The listing builds one solid part. Answer for the finished solid, in the listing's coordinates (mm). Face numbers are marked on the shaded views. A direction names the side the tool comes from. Give positions to 0.01 mm unless a question says otherwise; leave off trailing zeros. Write each loop counter-clockwise with the first axis right and the second up, starting at its lowest first coordinate (ties: lowest second). Pieces come first, ordered by that corner, then holes. Notation, with made-up numbers: (70.25, -32.5) - (113.25, -32.5) arc R21 cw to (113.25, -15.5) - close; hole circle Ø2 at (3.25, 56). An arc over 180 degrees is marked (long way). Answer as CSV lines item,"result". Start each with the question number.
(1) Find section B-B (x = -22). Write down the section's boundary in (y, z).
(2) Find section C-C (x = 102). Write down the section's boundary in (y, z).
(3) Find section A-A (y = -1079.5). Write down the section's boundary in (x, z).
(4) Straight lines are drawn through the part: probe 1 along Y at (x, z) = (-187.5, 29); probe 2 along Y at (x, z) = (-298, 49); probe 3 along Y at (x, z) = (-159, 67). For each, find the intervals that lie inside material, in ascending order.
(5) For a pull along X with two mould halves and no side action, classify the marked faces 3, 4 and 5 as pulls with the +X half, pulls with the -X half, needs draft (parallel to the pull), parting line crosses it, or undercut.
(6) Each of these flat-tipped pins is pushed along its axis until it touches: pin 1 Ø3 at (x, z) = (25, 78) entering from +Y; pin 2 Ø1.5 at (y, z) = (-348, 79) entering from -X; pin 3 Ø4 at (x, z) = (-44.5, 26) entering from +Y. Where does it stop, or does it pass through?
(7) For the marked faces 1 and 2, determine the directions among +Z, -Z, +X, -X, +Y, -Y from which every point of the face is accessible in a straight line to the end or side of a thin tool.
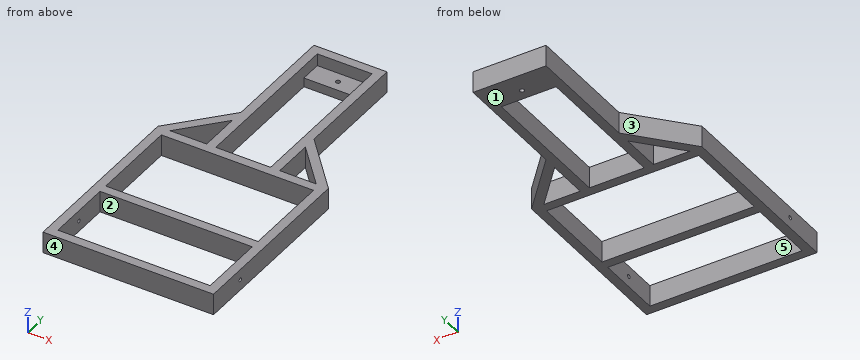
from build123d import *

# Parameters (mm, degrees)
F0_W          = 635
F0_H          = 38.1
F0_W_2        = 38.1
F1_DEPTH      = 88.9
F0_W_3        = 228.6
F0_H_2        = 88.9
F2_DEPTH      = 38.1
F3_R          = 9.525
F4_DEPTH      = 38.101
F5_R          = 7.9375
F6_DEPTH      = 673.101
F6_DEPTH_BACK = 38.101


with BuildPart() as f1:
    # F0 (on Top) → F1 (new body)
    with BuildSketch(Plane.XY):
        Polygon((0, -484.015493486), (0, 0), (-304.8, 0), (-304.8, -484.015493486), (-304.8, -541.165493486), (-304.8, -711.2), (-266.7, -711.2), (-266.7, -127), (-266.7, -38.1), (-38.1, -38.1), (-38.1, -127), (-38.1, -711.2), (0, -711.2), (0, -541.165493486), align=None)
        Polygon((-304.8, -541.165493486), (-304.8, -484.015493486), (-508, -711.2), (-456.8834860344, -711.2), align=None)
        Polygon((203.2, -711.2), (0, -484.015493486), (0, -541.165493486), (152.0834860344, -711.2), align=None)
        Polygon((203.2, -1117.6), (203.2, -711.2), (152.0834860344, -711.2), (0, -711.2), (-38.1, -711.2), (-152.4, -711.2), (-266.7, -711.2), (-304.8, -711.2), (-456.8834860344, -711.2), (-508, -711.2), (-508, -1117.6), (-469.9, -1117.6), (-469.9, -749.3), (165.1, -749.3), (165.1, -1117.6), align=None)
        with Locations((-152.4, -1136.65)):
            Rectangle(F0_W, F0_H)
        with Locations((184.15, -1136.65)):
            Rectangle(F0_W_2, F0_H)
        Polygon((203.2, -1473.2), (203.2, -1155.7), (165.1, -1155.7), (165.1, -1435.1), (-469.9, -1435.1), (-469.9, -1155.7), (-508, -1155.7), (-508, -1473.2), align=None)
        with Locations((-488.95, -1136.65)):
            Rectangle(F0_W_2, F0_H)
    extrude(amount=F1_DEPTH)

    # F0 (on Top) → F2 (join)
    with BuildSketch(Plane.XY):
        with Locations((-152.4, -82.55)):
            Rectangle(F0_W_3, F0_H_2)
    extrude(amount=F2_DEPTH)

    # F3 (on face) → F4 (cut, through all)
    with BuildSketch(Plane.XY.offset(38.1)):
        with Locations((-152.4, -82.55)):
            Circle(F3_R)
    extrude(amount=-F4_DEPTH, mode=Mode.SUBTRACT)

    # F5 (on face) → F6 (cut, two sides)
    with BuildSketch(Plane(origin=(165.1, 0, 0), x_dir=(0, -1, 0), z_dir=(-1, 0, 0))) as f6_sk:
        with Locations((1295.4, 44.45)):
            Circle(F5_R)
    extrude(amount=F6_DEPTH, mode=Mode.SUBTRACT)
    extrude(f6_sk.sketch, amount=-F6_DEPTH_BACK, mode=Mode.SUBTRACT)


solid = f1.part
Result set:
1,outline,"(-1473.2, 0) - (-1435.1, 0) - (-1435.1, 88.9) - (-1473.2, 88.9) - close; (-1155.7, 0) - (-1117.6, 0) - (-1117.6, 88.9) - (-1155.7, 88.9) - close; (-749.3, 0) - (0, 0) - (0, 88.9) - (-749.3, 88.9) - close"
2,outline,"(-1473.2, 0) - (-1435.1, 0) - (-1435.1, 88.9) - (-1473.2, 88.9) - close; (-1155.7, 0) - (-1117.6, 0) - (-1117.6, 88.9) - (-1155.7, 88.9) - close; (-749.3, 0) - (-711.2, 0) - (-711.2, 88.9) - (-749.3, 88.9) - close; (-655.2, 0) - (-598.05, 0) - (-598.05, 88.9) - (-655.2, 88.9) - close"
3,outline,"(-508, 0) - (-469.9, 0) - (-469.9, 88.9) - (-508, 88.9) - close; (165.1, 0) - (203.2, 0) - (203.2, 88.9) - (165.1, 88.9) - close"
4,probe 1,"-1473.2 to -1435.1, -1155.7 to -1117.6, -749.3 to -711.2, -127 to 0"
4,probe 2,"-1473.2 to -1435.1, -1155.7 to -1117.6, -749.3 to 0"
4,probe 3,"-1473.2 to -1435.1, -1155.7 to -1117.6, -749.3 to -711.2, -38.1 to 0"
5,face 3,"pulls with the -X half"
5,face 4,"needs draft"
5,face 5,"undercut"
6,pin 1,"y = -510.29"
6,pin 2,"x = -304.8"
6,pin 3,"y = 0"
7,face 1,"-Z, +X, -X, +Y, -Y"
7,face 2,"+Z, -Z"
